```python
from build123d import *

# Parameters (mm, degrees)
SKETCH2_W            = 38
SKETCH2_H            = 23.6
BOSS_EXTRUDE2_DEPTH  = 2.5
SKETCH3_W            = 35
SKETCH3_H            = 17.6
CUT_EXTRUDE2_DEPTH   = 2.5
SKETCH5_W            = 36.5
SKETCH5_H            = 2
SKETCH5_W_2          = 1.5
SKETCH5_H_2          = 19.6
BOSS_EXTRUDE3_DEPTH  = 26
SKETCH7_W            = 36.5
SKETCH7_H            = 2.5
BOSS_EXTRUDE5_DEPTH  = 1
SKETCH10_W           = 12.597499818
SKETCH10_H           = 2.5
SKETCH10_W_2         = 23.902500182
BOSS_EXTRUDE6_DEPTH  = 1
SKETCH11_W           = 2.5
SKETCH11_H           = 17.6
BOSS_EXTRUDE7_DEPTH  = 2
SKETCH15_W           = 30.589508609
SKETCH15_H           = 23.5
SKETCH15_W_2         = 3.8732763
CUT_EXTRUDE4_DEPTH   = 30
SKETCH16_W           = 3
SKETCH16_H           = 2.5
BOSS_EXTRUDE8_DEPTH  = 20
SKETCH17_W           = 3
SKETCH17_H           = 2.5
BOSS_EXTRUDE9_DEPTH  = 20
SKETCH19_W           = 5.5
SKETCH19_H           = 23.6
BOSS_EXTRUDE10_DEPTH = 16
SKETCH20_R           = 2.6
CUT_EXTRUDE6_DEPTH   = 30
SKETCH21_R           = 3.3
CUT_EXTRUDE7_DEPTH   = 0.8
SKETCH22_R           = 3.3
CUT_EXTRUDE8_DEPTH   = 0.8
FILLET1_R            = 5
FILLET3_R            = 5
SKETCH23_W           = 34.462784909
SKETCH23_H           = 2
BOSS_EXTRUDE11_DEPTH = 0.8
SKETCH24_W           = 34.462784909
SKETCH24_H           = 2
BOSS_EXTRUDE12_DEPTH = 0.8
SKETCH25_W           = 34.462784909
SKETCH25_H           = 2
BOSS_EXTRUDE13_DEPTH = 0.8
SKETCH26_W           = 34.462784909
SKETCH26_H           = 2
BOSS_EXTRUDE14_DEPTH = 0.8
CUT_EXTRUDE9_DEPTH   = 6


with BuildPart() as part:
    # Sketch2 → Boss-Extrude2 (new body)
    with BuildSketch(Plane.XY):
        with Locations((19, 11.8)):
            Rectangle(SKETCH2_W, SKETCH2_H)
    extrude(amount=BOSS_EXTRUDE2_DEPTH)

    # Sketch3 → Cut-Extrude2 (cut)
    with BuildSketch(Plane.XY.offset(2.5)):
        with Locations((20.5, 11.8)):
            Rectangle(SKETCH3_W, SKETCH3_H)
    extrude(amount=-CUT_EXTRUDE2_DEPTH, mode=Mode.SUBTRACT)

    # Sketch5 → Boss-Extrude3 (add)
    with BuildSketch(Plane.XY.offset(2.5)):
        with Locations((19.75, 22.6)):
            Rectangle(SKETCH5_W, SKETCH5_H)
        with Locations((0.75, 22.6)):
            Rectangle(SKETCH5_W_2, SKETCH5_H)
        with Locations((0.75, 11.8)):
            Rectangle(SKETCH5_W_2, SKETCH5_H_2)
        with Locations((0.75, 1)):
            Rectangle(SKETCH5_W_2, SKETCH5_H)
        with Locations((19.75, 1)):
            Rectangle(SKETCH5_W, SKETCH5_H)
    extrude(amount=BOSS_EXTRUDE3_DEPTH)

    # Sketch7 → Boss-Extrude5 (add)
    with BuildSketch(Plane(origin=(0, 2, 0), x_dir=(1, 0, 0), z_dir=(0, 1, 0))):
        with Locations((19.75, -27.25)):
            Rectangle(SKETCH7_W, SKETCH7_H)
    extrude(amount=BOSS_EXTRUDE5_DEPTH)

    # Sketch10 → Boss-Extrude6 (add)
    with BuildSketch(Plane.XZ.offset(-21.6)):
        with Locations((31.701250091, 27.25)):
            Rectangle(SKETCH10_W, SKETCH10_H)
        with Locations((13.451250091, 27.25)):
            Rectangle(SKETCH10_W_2, SKETCH10_H)
    extrude(amount=BOSS_EXTRUDE6_DEPTH)

    # Sketch11 → Boss-Extrude7 (add)
    with BuildSketch(Plane(origin=(1.5, 0, 0), x_dir=(0, 0, -1), z_dir=(1, 0, 0))):
        with Locations((-27.25, 11.8)):
            Rectangle(SKETCH11_W, SKETCH11_H)
    extrude(amount=BOSS_EXTRUDE7_DEPTH)

    # Sketch15 → Cut-Extrude4 (cut)
    with BuildSketch(Plane(origin=(0, 23.6, 0), x_dir=(1, 0, 0), z_dir=(0, 1, 0))):
        with Locations((18.831969395, -14.25)):
            Rectangle(SKETCH15_W, SKETCH15_H)
        with Locations((36.06336185, -14.25)):
            Rectangle(SKETCH15_W_2, SKETCH15_H)
    extrude(amount=-CUT_EXTRUDE4_DEPTH, mode=Mode.SUBTRACT)

    # Sketch16 → Boss-Extrude8 (add)
    with BuildSketch(Plane(origin=(0, 3, 0), x_dir=(1, 0, 0), z_dir=(0, 1, 0))):
        with Locations((36.5, -1.25)):
            Rectangle(SKETCH16_W, SKETCH16_H)
    extrude(amount=BOSS_EXTRUDE8_DEPTH)

    # Sketch17 → Boss-Extrude9 (add)
    with BuildSketch(Plane(origin=(0, 3, 0), x_dir=(1, 0, 0), z_dir=(0, 1, 0))):
        with Locations((36.5, -27.25)):
            Rectangle(SKETCH17_W, SKETCH17_H)
    extrude(amount=BOSS_EXTRUDE9_DEPTH)

    # Sketch19 → Boss-Extrude10 (add)
    with BuildSketch(Plane.ZY):
        with Locations((17, 11.8)):
            Rectangle(SKETCH19_W, SKETCH19_H)
        with Locations((11.5, 11.8)):
            Rectangle(SKETCH19_W, SKETCH19_H)
    extrude(amount=BOSS_EXTRUDE10_DEPTH)

    # Sketch20 → Cut-Extrude6 (cut)
    with BuildSketch(Plane(origin=(0, 23.6, 0), x_dir=(1, 0, 0), z_dir=(0, 1, 0))):
        with Locations((-8.54, -14.25)):
            Circle(SKETCH20_R)
    extrude(amount=-CUT_EXTRUDE6_DEPTH, mode=Mode.SUBTRACT)

    # Sketch21 → Cut-Extrude7 (cut)
    with BuildSketch(Plane(origin=(0, 23.6, 0), x_dir=(1, 0, 0), z_dir=(0, 1, 0))):
        with Locations((-8.54, -14.25)):
            Circle(SKETCH21_R)
    extrude(amount=-CUT_EXTRUDE7_DEPTH, mode=Mode.SUBTRACT)

    # Sketch22 → Cut-Extrude8 (cut)
    with BuildSketch(Plane.XZ):
        with Locations((-8.54, 14.25)):
            Circle(SKETCH22_R)
    extrude(amount=-CUT_EXTRUDE8_DEPTH, mode=Mode.SUBTRACT)

    # Fillet1
    fillet1_edges = [part.edges().sort_by_distance(p)[0] for p in [
        (-16, 11.8, 8.75),
    ]]
    fillet(fillet1_edges, radius=FILLET1_R)

    # Fillet3
    fillet3_edges = [part.edges().sort_by_distance(p)[0] for p in [
        (-16, 11.8, 19.75),
    ]]
    fillet(fillet3_edges, radius=FILLET3_R)

    # Sketch23 → Boss-Extrude11 (add)
    with BuildSketch(Plane(origin=(0, 0, 26), x_dir=(-1, 0, 0), z_dir=(0, 0, -1))):
        with Locations((-20.768607546, 22.6)):
            Rectangle(SKETCH23_W, SKETCH23_H)
    extrude(amount=BOSS_EXTRUDE11_DEPTH)

    # Sketch24 → Boss-Extrude12 (add)
    with BuildSketch(Plane.XY.offset(2.5)):
        with Locations((20.768607546, 22.6)):
            Rectangle(SKETCH24_W, SKETCH24_H)
    extrude(amount=BOSS_EXTRUDE12_DEPTH)

    # Sketch25 → Boss-Extrude13 (add)
    with BuildSketch(Plane(origin=(0, 0, 26), x_dir=(-1, 0, 0), z_dir=(0, 0, -1))):
        with Locations((-20.768607546, 1)):
            Rectangle(SKETCH25_W, SKETCH25_H)
    extrude(amount=BOSS_EXTRUDE13_DEPTH)

    # Sketch26 → Boss-Extrude14 (add)
    with BuildSketch(Plane.XY.offset(2.5)):
        with Locations((20.768607546, 1)):
            Rectangle(SKETCH26_W, SKETCH26_H)
    extrude(amount=BOSS_EXTRUDE14_DEPTH)

    # Sketch27 → Cut-Extrude9 (cut)
    with BuildSketch(Plane(origin=(1.5, 0, 0), x_dir=(0, 0, -1), z_dir=(1, 0, 0))):
        with BuildLine():
            ThreePointArc((-17.75, 11.8), (-16.724873734, 9.325126266), (-14.25, 8.3))
            Line((-14.25, 8.3), (-14.25, 11.8))
            Line((-14.25, 11.8), (-17.75, 11.8))
        make_face()
        with BuildLine():
            Line((-14.25, 11.8), (-14.25, 8.3))
            ThreePointArc((-14.25, 8.3), (-11.775126266, 9.325126266), (-10.75, 11.8))
            Line((-10.75, 11.8), (-14.25, 11.8))
        make_face()
        with BuildLine():
            Line((-17.75, 11.8), (-14.25, 11.8))
            Line((-14.25, 11.8), (-14.25, 15.3))
            ThreePointArc((-14.25, 15.3), (-16.724873734, 14.274873734), (-17.75, 11.8))
        make_face()
        with BuildLine():
            Line((-14.25, 15.3), (-14.25, 11.8))
            Line((-14.25, 11.8), (-10.75, 11.8))
            ThreePointArc((-10.75, 11.8), (-11.775126266, 14.274873734), (-14.25, 15.3))
        make_face()
    extrude(amount=-CUT_EXTRUDE9_DEPTH, mode=Mode.SUBTRACT)


solid = part.part
```
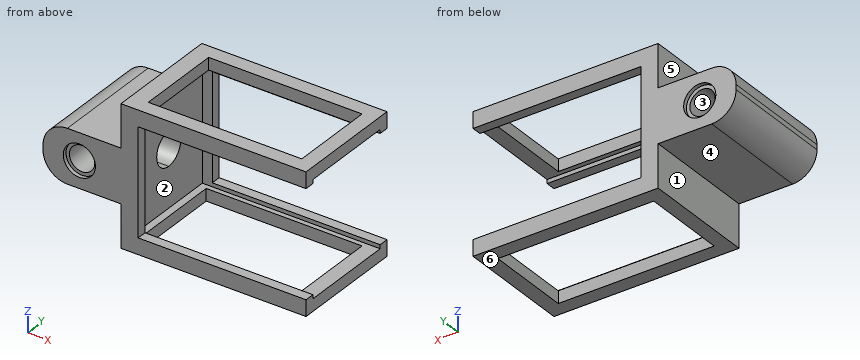
Can you work these out from the model? Positions are in its coordinate system, mm. Face numbers are marked on the shaded views. A direction names the side the tool comes from. Round coordinates to 2 decimals unless told otherwise and drop trailing zeros. Loops run counter-clockwise (first coordinate to the right, second up) from the corner with the lowest first, then second, coordinate; pieces in that order, holes last. Notation, with made-up numbers: M 53.5,-4.75 L 57.5,-4.75 A28 ccw 57.5,30.25 Z; hole C 46.25,-24 d5. An arc over 180 degrees is marked long. Answer in a Markdown table with one row per item.
1. On a 3-axis mill with a long thin cutter (end or side, diameter ignored), from which of +Z, -Z, +X, -X, +Y, -Y can I reach the whole of each face in a straight line? I mean the marked faces 5 and 6. Say none if no direction works.
Established:
| item | result |
|---|---|
| face 5 | +Z, -X, +Y, -Y |
| face 6 | -Z, +X, -X, +Y, -Y |
2. If we section it at C-C, the plane x = 8: Please give me the cut outline in (y, z).
Established:
| item | result |
|---|---|
| outline | M 0,0 L 3,0 L 3,2.5 L 2,2.5 L 2,3.3 L 0,3.3 Z; M 0,25.2 L 2,25.2 L 2,26 L 3,26 L 3,28.5 L 0,28.5 Z; M 20.6,0 L 23.6,0 L 23.6,3.3 L 21.6,3.3 L 21.6,2.5 L 20.6,2.5 Z; M 20.6,26 L 21.6,26 L 21.6,25.2 L 23.6,25.2 L 23.6,28.5 L 20.6,28.5 Z |
3. Thinking about a two-plate mould opening in X: for the marked faces 1, 2, 3 and 4, which applies, pulls with the +X half, pulls with the -X half, needs draft (parallel to the pull), parting line crosses it, or undercut?
Established:
| item | result |
|---|---|
| face 1 | pulls with the -X half |
| face 2 | pulls with the +X half |
| face 3 | undercut |
| face 4 | needs draft |
4. Please list where these lines run through material, in increasing order: line 1 (Y direction, x = 20, z = 1.5); line 2 (X direction, y = 13, z = 14.25); line 3 (Z direction, x = -8.54, y = 5.5). Write a range as from..to.
Established:
| item | result |
|---|---|
| line 1 | 0..3, 20.6..23.6 |
| line 2 | -16..-11.14, -5.94..-4.5 |
| line 3 | 8.75..11.65, 16.85..19.75 |
5. I'm going to push flat-ended pins straight in: pin 1 Ø1.6 at (y, z) = (22.5, 10) entering from +X; pin 2 Ø3 at (y, z) = (9.5, 27.5) entering from -X; pin 3 Ø8.5 at (x, z) = (-8.54, 14.25) entering from -Y; pin 4 Ø1.5 at (y, z) = (11.5, 21.5) entering from +X. Where does each tip first touch, or does it pass through?
Established:
| item | result |
|---|---|
| pin 1 | x = 3.54 |
| pin 2 | x = 0 |
| pin 3 | y = 0 |
| pin 4 | x = 1.5 |
6. If we section it at D-D, the plane z = 8: Please give me the cut outline in (x, y), plus the area to 3 significant figures.
Established:
| item | result |
|---|---|
| outline | M 0,0 L 3.54,0 L 3.54,2 L 1.5,2 L 1.5,21.6 L 3.54,21.6 L 3.54,23.6 L 0,23.6 Z |
| area | 43.5 mm² |
7. If we section it at A-A, the plane x = -8.54: Please give me the cut outline in (y, z), plus the area to 3 significant figures.
Established:
| item | result |
|---|---|
| outline | M 0,8.75 L 23.6,8.75 L 23.6,10.95 L 22.8,10.95 L 22.8,11.65 L 0.8,11.65 L 0.8,10.95 L 0,10.95 Z; M 0,17.55 L 0.8,17.55 L 0.8,16.85 L 22.8,16.85 L 22.8,17.55 L 23.6,17.55 L 23.6,19.75 L 0,19.75 Z |
| area | 135 mm² |
8. If we section it at B-B, the plane y = 9.25: Please give me the cut outline in (x, z), plus the area to 3 significant figures.
Established:
| item | result |
|---|---|
| outline | M -16,13.75 A5 ccw -11,8.75 L 0,8.75 L 0,0 L 3,0 L 3,2.5 L 1.5,2.5 L 1.5,11.85 L -4.5,11.85 L -4.5,16.65 L 1.5,16.65 L 1.5,26 L 3.5,26 L 3.5,28.5 L 0,28.5 L 0,19.75 L -11,19.75 A5 ccw -16,14.75 Z; M 35,0 L 38,0 L 38,2.5 L 35,2.5 Z; M 35,26 L 38,26 L 38,28.5 L 35,28.5 Z; hole C -8.54,14.25 d5.2 |
| area | 182 mm² |
